Part model, mm, in its own coordinate system. Face numbers are marked on the shaded views. A direction names the side the tool comes from. Round coordinates to 2 decimals unless told otherwise and drop trailing zeros. Order: outer loops, then holes, each group sorted by start corner. A loop starts at its lowest first (then second) coordinate and runs counter-clockwise, first axis right, second up. Notation, with made-up numbers: M 38,54 L 62,54 A13 cw 62,61 Z; hole C -37.5,38 d5. An arc over 180 degrees is marked long. Write each question's results on one line, items separated by ' | '. Start each with the question number.
1. Which spindle directions (+Z, -Z, +X, -X, +Y, -Y) get a long thin tool onto all of the face, cutting with end or side? Do the marked faces 4, 5, 6, 7 and 8. Say none if no direction does.
2. Band-saw the part on C-C, the plane x = 12.5. List the corners of the cut face in (y, z).
3. Band-saw the part on B-B, the plane z = -28.5. List the corners of the cut face in (x, y).
4. Band-saw the part on D-D, the plane z = 79. List the corners of the cut face in (x, y), then the cut area to 3 significant figures.
5. Two-plate mould, pull along Z, no slides. Class the marked faces 1, 2 and 3: +Z half, -Z half, draft (parallel to the pull), parting line (faces both ways), or undercut.
6. Band-saw the part on A-A, the plane y = -18.25. List the corners of the cut face in (x, z), then the cut area to 3 significant figures.
7. Drop flat-ended pins along their axis: pin 1 Ø1 at (x, y) = (-11.5, -10.5) entering from +Z; pin 2 Ø5 at (x, z) = (19.5, 68) entering from +Y; pin 3 Ø1 at (x, y) = (-7.5, -4.5) entering from -Z (3 decimals). Give the stop position or say it passes through.
8. Probe L1, parallel to X at y = -21.5, z = -9; L2, parallel to Y at x = 27.5, z = 6; L3, parallel to Z at x = 23.5, y = -14. List the from-to ranges inside material, lowest first. Write a range as [from, to].
```python
from build123d import *

# Parameters (mm, degrees)
F0_W     = 58.329247
F0_H     = 100.166194
F1_DEPTH = 25.4
F3_D     = 38.1
F5_W     = 22.291495
F5_H     = 12.931229
F6_DEPTH = 25.4
F8_W     = 57.983957
F8_H     = 36.597609
F9_DEPTH = 12.285994
F10_R    = 7.926633


with BuildPart() as f1:
    # F0 (on Front) → F1 (new body)
    with BuildSketch(Plane.XZ):
        with Locations((0.23458, 8.289784)):
            Rectangle(F0_W, F0_H)
    extrude(amount=F1_DEPTH)

    # F3 (through all)
    with Locations(Plane.XZ.offset(25.4)):
        with Locations((0.23458, -41.793313)):
            Hole(F3_D / 2)

    # F5 (on face) → F6 (join)
    with BuildSketch(Plane.XY.offset(58.372881)):
        with Locations((-1.115124, -10.430084)):
            Rectangle(F5_W, F5_H)
    extrude(amount=F6_DEPTH)

    # F8 (on face) → F9 (join)
    with BuildSketch(Plane.XZ.offset(16.895698)):
        with Locations((-1.133726, 85.148781)):
            Rectangle(F8_W, F8_H)
    extrude(amount=F9_DEPTH)

    # F10
    f10_edges = [f1.edges().sort_by_distance(p)[0] for p in [
        (27.858253, -29.181693, 85.148782),
        (-1.133725, -29.181693, 103.447586),
        (-1.133725, -29.181693, 66.849977),
        (-30.125704, -29.181693, 85.148782),
    ]]
    fillet(f10_edges, radius=F10_R)


solid = f1.part
```
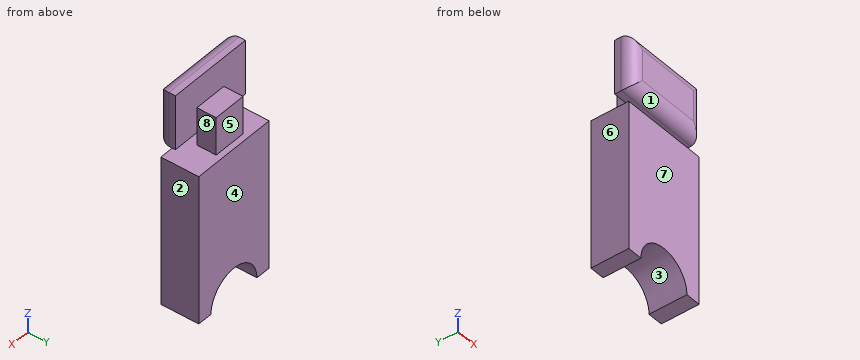
Solution:
1) face 4: +Z, -Z, +X, -X, +Y | face 5: +Z, +X, -X, +Y | face 6: -Z, -X, +Y, -Y | face 7: -Z, +X, -X, -Y | face 8: +Z, +X, +Y
2) outline: M -29.18,74.78 A7.93 ccw -21.26,66.85 L -16.9,66.85 L -16.9,103.45 L -21.26,103.45 A7.93 ccw -29.18,95.52 Z; M -25.4,-27.22 L 0,-27.22 L 0,58.37 L -25.4,58.37 Z
3) outline: M -28.93,-25.4 L -13.41,-25.4 L -13.41,0 L -28.93,0 Z; M 13.88,-25.4 L 29.4,-25.4 L 29.4,0 L 13.88,0 Z
4) outline: M -30.13,-21.26 A7.93 ccw -22.2,-29.18 L 19.93,-29.18 A7.93 ccw 27.86,-21.26 L 27.86,-16.9 L 10.03,-16.9 L 10.03,-3.96 L -12.26,-3.96 L -12.26,-16.9 L -30.13,-16.9 Z | area: 974 mm^2
5) face 1: undercut | face 2: draft | face 3: -Z half
6) outline: M -30.13,66.85 L 27.86,66.85 L 27.86,103.45 L -30.13,103.45 Z; M -28.93,-41.79 L -18.82,-41.79 A19.05 cw 19.28,-41.79 L 29.4,-41.79 L 29.4,58.37 L -28.93,58.37 Z | area: 7,390 mm^2
7) pin 1: z = 83.77 | pin 2: y = -16.9 | pin 3: z = -24.615
8) L1: [-28.93, 29.4] | L2: [-25.4, 0] | L3: [-41.79, 58.37]
